The drawing under review shows one solid part. Ordinate dimensions are in mm from its lowest x, y, z. A direction names the side the tool comes from. Coordinates: 2 decimals unless noted, no trailing zeros. Order: outer loops, then holes, each group sorted by start corner. A loop starts at its lowest first (then second) coordinate and runs counter-clockwise, first axis right, second up. Notation, with made-up numbers: (53, 35) -> (94, 35) arc R24 ccw to (94, 67) -> close; hole circle Ø8 at (26.25, 51.25). An arc over 180 degrees is marked (long way). Use one line per item in the form item = value.
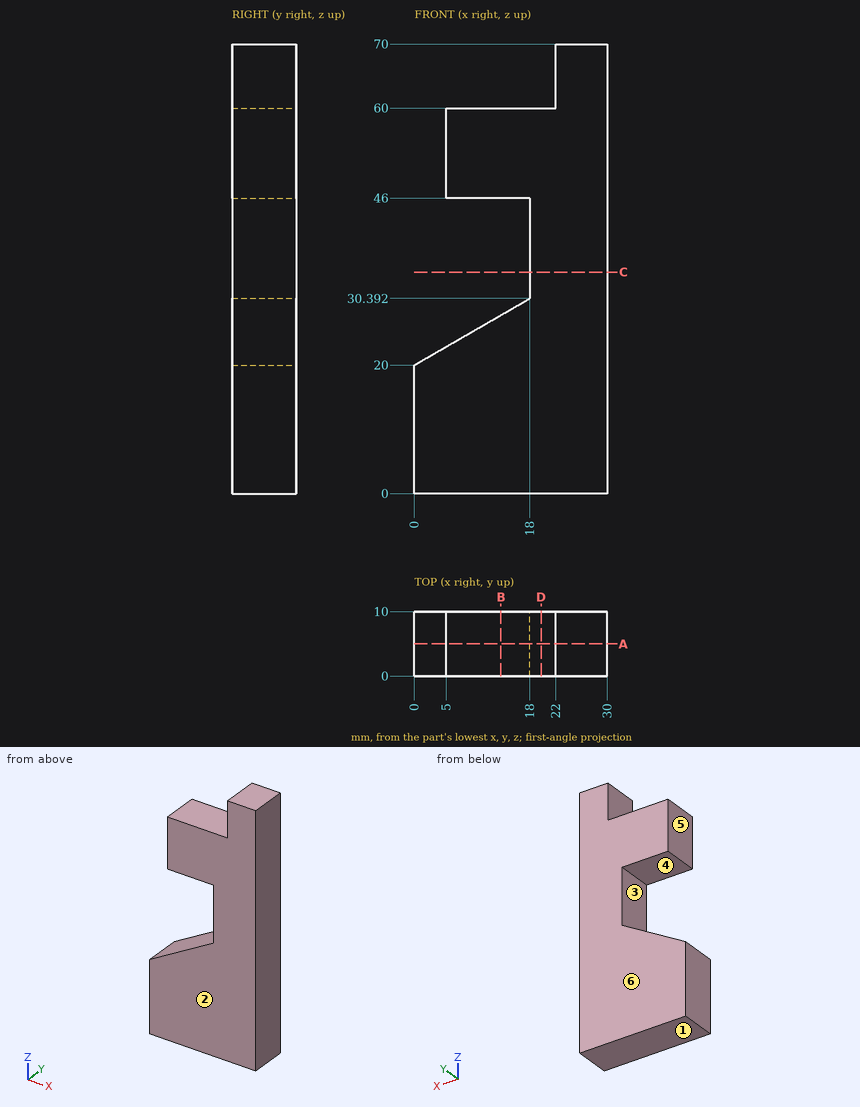
Item 1: Draft analysis for pull direction Z (two halves, no side actions). For the marked faces 1, 2, 3 and 4, state which applies: released by +Z, released by -Z, zero draft, split by the parting line, or undercut.
Results found:
face_1 = released by -Z
face_2 = zero draft
face_3 = undercut
face_4 = undercut
Item 2: Clearance check with a flat-ended pin moving along its axis: pin 1 (5 mm diameter, centred on x = 14, y = 7.5, fed in from +Z). State where the tip first meets the part, or that it passes through.
Results found:
pin_1 = 60
Item 3: We need section C-C (z = 34.5). Write out the cut boundary in (x, y), plus the area to 3 significant figures.
Results found:
outline = (18, 0) -> (30, 0) -> (30, 10) -> (18, 10) -> close
area = 120 mm²
Item 4: We need section D-D (x = 19.75). Write out the cut boundary in (y, z), plus the area to 3 significant figures.
Results found:
outline = (0, 0) -> (10, 0) -> (10, 60) -> (0, 60) -> close
area = 600 mm²
Item 5: To check wall thickness, follow L1, parallel to X at y = 7, z = 64; L2, parallel to Z at x = 10.5, y = 3; L3, parallel to Z at x = 20, y = 8. State the ranges of each line that lie inside material, in increasing order. Write a range as from..to.
Results found:
L1 = 22..30
L2 = 0..26.06, 46..60
L3 = 0..60
Item 6: We need section A-A (y = 5). Write out the cut boundary in (x, z).
Results found:
outline = (0, 0) -> (30, 0) -> (30, 70) -> (22, 70) -> (22, 60) -> (5, 60) -> (5, 46) -> (18, 46) -> (18, 30.39) -> (0, 20) -> close
Item 7: We need section B-B (x = 13.5). Write out the cut boundary in (y, z).
Results found:
outline = (0, 0) -> (10, 0) -> (10, 27.79) -> (0, 27.79) -> close; (0, 46) -> (10, 46) -> (10, 60) -> (0, 60) -> close
Item 8: Tool access review of the marked faces 5 and 6: name each direction out of +Z, -Z, +X, -X, +Y, -Y from which nothing blocks a thin tool from reaching the whole face with its end or side.
Results found:
face_5 = +Z, -X, +Y, -Y
face_6 = +Z, -Z, +X, -X, +Y
